Autodesk Inventor part; units mm, degrees
ref_plane "YZ Plane" through (0, 0, 0) normal (1, 0, 0) x (0, 1, 0)
ref_plane "XZ Plane" through (0, 0, 0) normal (0, 1, 0) x (-1, 0, 0)
ref_plane "XY Plane" through (0, 0, 0) normal (0, 0, 1) x (1, 0, 0)
sketch "Sketch1" plane through (0, 0, 0) normal (0, 0, 1) x (1, 0, 0)
  circle A0 centre (0, 0) radius 15
  circle A1 centre (208.6498, 0) radius 15
  line L0 (0, 15) -> (208.6498, 15)
  line L1 (208.6498, -15) -> (0, -15)
  line L2 (208.6498, 15) -> (221.6402, 7.5)
  line L3 (221.6402, 7.5) -> (221.6402, -7.5)
  line L4 (221.6402, -7.5) -> (208.6498, -15)
  point P0 (208.6498, -15)
  dimension "d0" = 30
  dimension "d1" = 208.6498
  dimension "d16" = 180
extrude "Extrusion1" add sketch "Sketch1" along normal blind 20 contours A0 | A0 L0 A1 L1 | L2 L3 L4 A1
sketch "Sketch2" plane through (0, 0, 0) normal (0, 0, -1) x (-1, 0, 0)
  circle A0 centre (-208.6498, 0) radius 3.75
  circle A1 centre (-167.7787, 0) radius 3.75
  line L0 (-210.8998, 3) -> (-165.5287, 3)
  line L1 (-210.8998, -3) -> (-165.5287, -3)
  line L2 (63.328, 0) -> (-274.9682, 0)
  line L3 (-221.6402, -7.5) -> (-221.6402, 7.5)
  point P0 (0, 0)
  point P1 (-170.0287, 3)
  point P2 (-170.0287, -3)
  point P3 (-206.3998, 3)
  point P4 (-206.3998, -3)
  point P5 (-208.6498, 15)
  point P6 (-221.6402, 0)
  dimension "d7" = 7.5
  dimension "d8" = 40.8711
  dimension "d11" = 6
extrude "Extrusion2" add sketch "Sketch2" along normal blind 30 contours L2 A0 L0 | A0 L1 L2 | L2 A1 L1 | A1 L0 L2
sketch "Sketch3" plane through (0, 0, 0) normal (0, 0, -1) x (-1, 0, 0)
  arc A0 (-210.8998, 3) -> (-210.8998, -3) centre (-208.6498, 0) ccw
  point P0 (0, 0)
  point P1 (-20, 0)
  dimension "d18" = 188.6498
hole "Hole1" at (20, 0, 0) direction (0, 0, 1) diameter 14 end through all
sketch "Sketch5" plane through (0, 0, 20) normal (0, 0, 1) x (1, 0, 0)
  circle A0 centre (20, 0) radius 7
  point P0 (0, 0)
  point P1 (13, 0)
  dimension "d34" = 7
hole "Hole3" at (13, 0, 20) direction (0, 0, -1) diameter 38 depth 15
sketch "Sketch6" plane through (1.3381, -15, 5) normal (0, 0, 1) x (1, 0, 0)
  arc A0 (23.3238, 0) -> (23.3238, 30) centre (11.6619, 15) ccw construction
  line L0 (30.6619, 15) -> (-7.3381, 15) construction
  arc A1 (0, 30) -> (0, 0) centre (11.6619, 15) ccw construction
  circle A2 centre (11.6619, 15) radius 15.5 construction
  point P0 (-1.3381, 15)
  point P1 (25.0853, 22.75)
  point P2 (25.0853, 7.25)
  point P3 (-1.7615, 22.75)
  point P4 (-1.7615, 7.25)
  dimension "d42" = 15.5
  dimension "d43" = 31
  dimension "d44" = 15.5
hole "Hole4" at (26.4234, 7.75, 5) at (26.4234, -7.75, 5) at (-0.4234, 7.75, 5) at (-0.4234, -7.75, 5) direction (0, 0, -1) diameter 4 end through all
sketch "Sketch7" plane through (0, 0, -30) normal (0, 0, -1) x (-1, 0, 0)
  line L0 (-165.5287, 3) -> (-170.0287, 3)
  arc A0 (-170.0287, 3) -> (-170.0287, -3) centre (-167.7787, 0) ccw
  line L1 (-170.0287, -3) -> (-165.5287, -3)
  arc A1 (-165.5287, -3) -> (-165.5287, 3) centre (-167.7787, 0) ccw
  point P0 (0, 0)
extrude "Extrusion3" add sketch "Sketch7" along normal blind 5
properties part number "LOWER_LINKAGE" material "ABS Plastic"
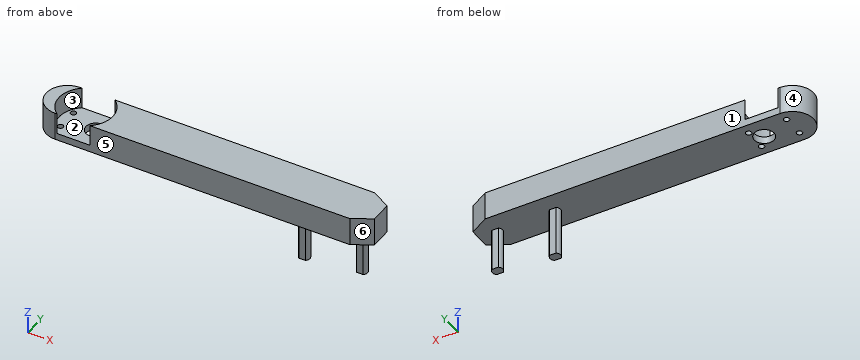
Source: CAD feature listing. Evaluate the final solid. Frame: model axes, mm. Face numbers are marked on the shaded views. A direction names the side the tool comes from. Give positions to 0.01 mm unless a question says otherwise; leave off trailing zeros. Write each loop counter-clockwise with the first axis right and the second up, starting at its lowest first coordinate (ties: lowest second). Pieces come first, ordered by that corner, then holes. Notation, with made-up numbers: M 44,5.25 L 63,5.25 A31 ccw 63,36.25 Z; hole C 61.25,-38.5 d6. An arc over 180 degrees is marked long. Return JSON: item names as keys, results as strings. Group by question number.
1) Cut plane C-C, the plane y = 0. Output: boundary loops of the cut face in (x, z), plus the area to 3 significant figures.
2) Cut plane A-A, the plane x = 20. Output: boundary loops of the cut face in (y, z).
3) Cut plane D-D, the plane x = 168. Output: boundary loops of the cut face in (y, z), plus the area to 3 significant figures.
4) Set-up query: the marked faces 1 and 2. Return all of +Z, -Z, +X, -X, +Y, -Y with unobstructed straight access to the full face (end or side cutting, diameter ignored); none if empty.
5) Pull-direction query (X, two-part tool) for the marked faces 3, 4, 5 and 6; classes: pulls with the +X half, pulls with the -X half, needs draft (parallel to the pull), parting line crosses it, or undercut.
6) Material intervals for line 1 along X through (y, z) = (-7.75, 1.3); line 2 along Z through (x, y) = (128, -4.5); line 3 along Y through (x, z) = (208, -28.5), sorted ascending. Write a range as [from, to].
7) Pin query (flat end, axial travel): P1, Ø3.5, axis at x = 168, z = -16, coming from the -Y side; P2, Ø5, axis at y = 3, z = 1.5, coming from the -X side; P3, Ø3.5, axis at x = 208, z = -17, coming from the +Y side; P4, Ø3.5, axis at x = 26.42, y = 7.75, coming from the -Z side. Return the tip coordinate at first contact, or that it passes through.
8) Cut plane B-B, the plane z = -6.5. Output: boundary loops of the cut face in (x, y).
Recorded:
{
 "1": {"outline": "M -15,0 L 13,0 L 13,5 L -6,5 L -6,20 L -15,20 Z; M 27,0 L 164.03,0 L 164.03,-35 L 171.53,-35 L 171.53,0 L 204.9,0 L 204.9,-30 L 212.4,-30 L 212.4,0 L 221.64,0 L 221.64,20 L 32,20 L 32,5 L 27,5 Z", "area": "4,580 mm²"},
 "2": {"outline": "M -15,0 L -7,0 L -7,5 L -15,5 Z; M 7,0 L 15,0 L 15,5 L 7,5 Z"},
 "3": {"outline": "M -15,0 L -3,0 L -3,-35 L 3,-35 L 3,0 L 15,0 L 15,20 L -15,20 Z", "area": "810 mm²"},
 "4": {"face 1": "+Z, -Z, +X, -X, +Y", "face 2": "+Z"},
 "5": {"face 3": "undercut", "face 4": "pulls with the -X half", "face 5": "needs draft", "face 6": "pulls with the +X half"},
 "6": {"line 1": "x = [-12.84, -2.42], [1.58, 24.42], [28.42, 221.21]", "line 2": "z = [0, 20]", "line 3": "y = [-3, 3]"},
 "7": {"P1": "stops at y = -3", "P2": "stops at x = -14.99", "P3": "stops at y = 3", "P4": "passes through"},
 "8": {"outline": "M 165.53,-3 L 170.03,-3 A3.75 ccw 170.03,3 L 165.53,3 A3.75 ccw Z; M 206.4,-3 L 210.9,-3 A3.75 ccw 210.9,3 L 206.4,3 A3.75 ccw Z"}
}
